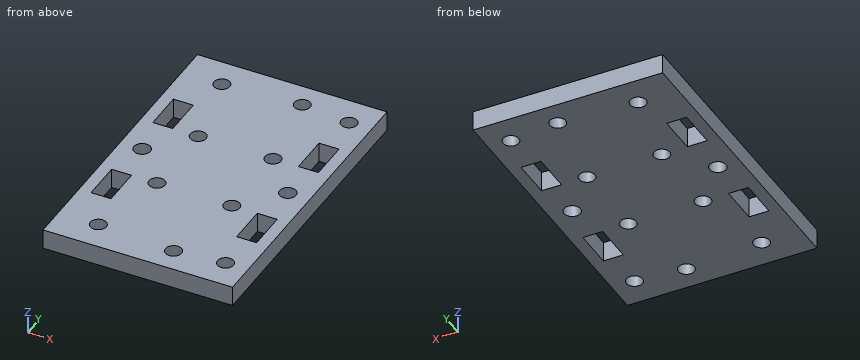
Autodesk Inventor part; units mm, degrees
ref_plane "YZ Plane" through (0, 0, 0) normal (1, 0, 0) x (0, 1, 0)
ref_plane "XZ Plane" through (0, 0, 0) normal (0, 1, 0) x (-1, 0, 0)
ref_plane "XY Plane" through (0, 0, 0) normal (0, 0, 1) x (1, 0, 0)
sketch "Эскиз1" plane through (0, 0, 0) normal (0, 0, 1) x (1, 0, 0)
  circle A0 centre (-7.5, -6.95) radius 1.5 construction
  circle A1 centre (7.5, -6.95) radius 1.5 construction
  circle A2 centre (-7.5, -22.95) radius 1.5 construction
  circle A3 centre (7.5, -22.95) radius 1.5 construction
  circle A4 centre (-7.5, -6.95) radius 1.6
  circle A5 centre (7.5, -6.95) radius 1.6
  circle A6 centre (7.5, -22.95) radius 1.6
  circle A7 centre (-7.5, -22.95) radius 1.6
  line L0 (-7.5, -6.95) -> (7.5, -22.95) construction
  line L1 (-19, 15.05) -> (19, 15.05)
  line L2 (19, 15.05) -> (19, -44.95)
  line L3 (19, -44.95) -> (-19, -44.95)
  line L4 (-19, -44.95) -> (-19, 15.05)
  line L5 (-19, 15.05) -> (19, -44.95) construction
  line L6 (19, 15.05) -> (-19, -44.95) construction
  point P0 (0, 0)
  point P1 (0, -14.95)
  dimension "d0" = 3.2
  dimension "d1" = 3.2
  dimension "d2" = 3.2
  dimension "d3" = 3.2
  dimension "d4" = 38
  dimension "d5" = 60
extrude "Выдавливание1" add sketch "Эскиз1" along normal blind 4
sketch "Эскиз2" plane through (0, 0, 4) normal (0, 0, 1) x (1, 0, 0)
  circle A0 centre (-7.5, -22.95) radius 1.6 construction
  circle A1 centre (7.5, -6.95) radius 1.6 construction
  circle A2 centre (7.5, -6.95) radius 1.6 construction
  line L0 (-7.5, -22.95) -> (7.5, -6.95) construction
  line L1 (16.6, -30.95) -> (-16.6, -30.95) construction
  line L2 (-16.6, -30.95) -> (-16.6, 1.05) construction
  line L3 (-16.6, 1.05) -> (16.6, 1.05) construction
  line L4 (16.6, 1.05) -> (16.6, -30.95) construction
  line L5 (16.6, -30.95) -> (-16.6, 1.05) construction
  line L6 (-16.6, -30.95) -> (16.6, 1.05) construction
  line L7 (-16.6, -30.95) -> (-12.6, -30.95)
  line L8 (-12.6, -30.95) -> (-12.6, -22.95)
  line L9 (-12.6, -22.95) -> (-16.6, -22.95)
  line L10 (-16.6, -22.95) -> (-16.6, -30.95)
  line L11 (-16.6, 1.05) -> (-12.6, 1.05)
  line L12 (-12.6, 1.05) -> (-12.6, -6.95)
  line L13 (-12.6, -6.95) -> (-16.6, -6.95)
  line L14 (-16.6, -6.95) -> (-16.6, 1.05)
  line L15 (16.6, -30.95) -> (12.6, -30.95)
  line L16 (12.6, -30.95) -> (12.6, -22.95)
  line L17 (12.6, -22.95) -> (16.6, -22.95)
  line L18 (16.6, -22.95) -> (16.6, -30.95)
  line L19 (16.6, 1.05) -> (12.6, 1.05)
  line L20 (12.6, 1.05) -> (12.6, -6.95)
  line L21 (12.6, -6.95) -> (16.6, -6.95)
  line L22 (16.6, -6.95) -> (16.6, 1.05)
  point P0 (0, -14.95)
  dimension "d41" = 33.2
  dimension "d42" = 32
  dimension "d43" = 4
  dimension "d44" = 8
  dimension "d45" = 4
  dimension "d46" = 8
  dimension "d47" = 4
  dimension "d48" = 4
  dimension "d49" = 8
  dimension "d50" = 8
extrude "Выдавливание2" cut sketch "Эскиз2" against normal blind 4
sketch "Эскиз3" plane through (0, 0, 4) normal (0, 0, 1) x (1, 0, 0)
  line L0 (12.6, -22.95) -> (16.6, -22.95) construction
  line L1 (16.6, -6.95) -> (12.6, -6.95) construction
  line L2 (14.6, -22.95) -> (14.6, -6.95) construction
  circle A0 centre (14.6, -14.95) radius 1.65
  line L3 (-19, -44.95) -> (19, -44.95)
  line L4 (0, -44.95) -> (0, 15.05) construction
  line L5 (19, 15.05) -> (-19, 15.05)
  circle A1 centre (-14.6, -14.95) radius 1.65
  point P0 (0, 0)
  dimension "d18" = 3.3
extrude "Выдавливание3" cut sketch "Эскиз3" against normal blind 10
sketch "Эскиз4" plane through (0, 0, 4) normal (0, 0, 1) x (1, 0, 0)
  line L0 (19, -44.95) -> (19, 15.05)
  line L1 (19, -14.95) -> (-2.8531, -14.95) construction
  line L2 (4.6, -39.95) -> (4.6, 10.05) construction
  circle A0 centre (4.6, -39.95) radius 1.6
  circle A1 centre (4.6, 10.05) radius 1.6
  point P0 (0, 0)
  point P1 (4.6, -14.95)
  dimension "d22" = 50
  dimension "d24" = 3.2
  dimension "d25" = 3.2
extrude "Выдавливание4" cut sketch "Эскиз4" against normal blind 10
sketch "Эскиз5" plane through (0, 0, 4) normal (0, 0, 1) x (1, 0, 0)
  line L0 (16.6, -30.95) -> (12.6, -30.95) construction
  line L1 (16.6, 1.05) -> (12.6, 1.05) construction
  line L2 (-12.6, 1.05) -> (-16.6, 1.05) construction
  line L3 (-12.6, -30.95) -> (-16.6, -30.95) construction
  circle A0 centre (14.5, -38.95) radius 1.6
  line L4 (19, -44.95) -> (19, 15.05)
  line L5 (19, -14.95) -> (-19, -14.95) construction
  line L6 (-19, 15.05) -> (-19, -44.95)
  line L7 (19, 15.05) -> (-19, 15.05)
  line L8 (0, 15.05) -> (0, -44.95) construction
  line L9 (-19, -44.95) -> (19, -44.95)
  circle A1 centre (14.5, 9.05) radius 1.6
  line L10 (0, -44.95) -> (0, 15.05) construction
  line L11 (-16.6, -30.95) -> (-12.6, -30.95) construction
  line L12 (-16.6, 1.05) -> (-12.6, 1.05) construction
  circle A2 centre (-11, -38.95) radius 1.6
  circle A3 centre (-11, 9.05) radius 1.6
  point P0 (0, 0)
  dimension "d28" = 3.2
  dimension "d33" = 3.2
  dimension "d34" = 3.2
  dimension "d35" = 6
  dimension "d36" = 6
  dimension "d37" = 8
  dimension "d38" = 8
  dimension "d39" = 6
  dimension "d40" = 4.5
extrude "Выдавливание5" cut sketch "Эскиз5" against normal blind 10 contours A0 | A1 | A2 | A3
properties part number "пол_каретки"
Work out the finished part from the listing and answer in its coordinate system (mm). Round coordinates to 2 decimals unless told otherwise and drop trailing zeros. Order: outer loops, then holes, each group sorted by start corner. A loop starts at its lowest first (then second) coordinate and runs counter-clockwise, first axis right, second up. Notation, with made-up numbers: M 47.5,88 L 53.5,88 A14 ccw 53.5,94 Z; hole C -4,73 d3. An arc over 180 degrees is marked long. Put each result on its own line as item: value. Start each with the question number.
Q1. Section C-C, the plane y = -2 is taken. Write down the section's boundary in (x, z), and give its area (3 significant figures).
Q2. Section A-A, the plane z = 1.4 is taken. Give the number of separate pieces and of enclosed holes in the cut face, and give its area (3 significant figures).
Q3. Section D-D, the plane x = 15 is taken. Write down the section's boundary in (y, z).
Q4. Section B-B, the plane x = 7.5 is taken. Write down the section's boundary in (y, z).
Q5. Straight lines are drawn through the part: L1, parallel to Y at x = 7.5, z = 2.3; L2, parallel to X at y = -27, z = 3.7; L3, parallel to X at y = -7, z = 3.1. For each, find the intervals that lie inside material, in ascending order. Write a range as [from, to].
Findings below:
1. outline: M -19,0 L -16.6,0 L -16.6,4 L -19,4 Z; M -12.6,0 L 12.6,0 L 12.6,4 L -12.6,4 Z; M 16.6,0 L 19,0 L 19,4 L 16.6,4 Z
1. area: 120 mm^2
2. separate pieces: 1
2. enclosed holes: 16
2. area: 2,050 mm^2
3. outline: M -44.95,0 L -40.47,0 L -40.47,4 L -44.95,4 Z; M -37.43,0 L -30.95,0 L -30.95,4 L -37.43,4 Z; M -22.95,0 L -16.55,0 L -16.55,4 L -22.95,4 Z; M -13.35,0 L -6.95,0 L -6.95,4 L -13.35,4 Z; M 1.05,0 L 7.53,0 L 7.53,4 L 1.05,4 Z; M 10.57,0 L 15.05,0 L 15.05,4 L 10.57,4 Z
4. outline: M -44.95,0 L -24.55,0 L -24.55,4 L -44.95,4 Z; M -21.35,0 L -8.55,0 L -8.55,4 L -21.35,4 Z; M -5.35,0 L 15.05,0 L 15.05,4 L -5.35,4 Z
5. L1: y = [-44.95, -24.55], [-21.35, -8.55], [-5.35, 15.05]
5. L2: x = [-19, -16.6], [-12.6, 12.6], [16.6, 19]
5. L3: x = [-19, -9.1], [-5.9, 5.9], [9.1, 19]
